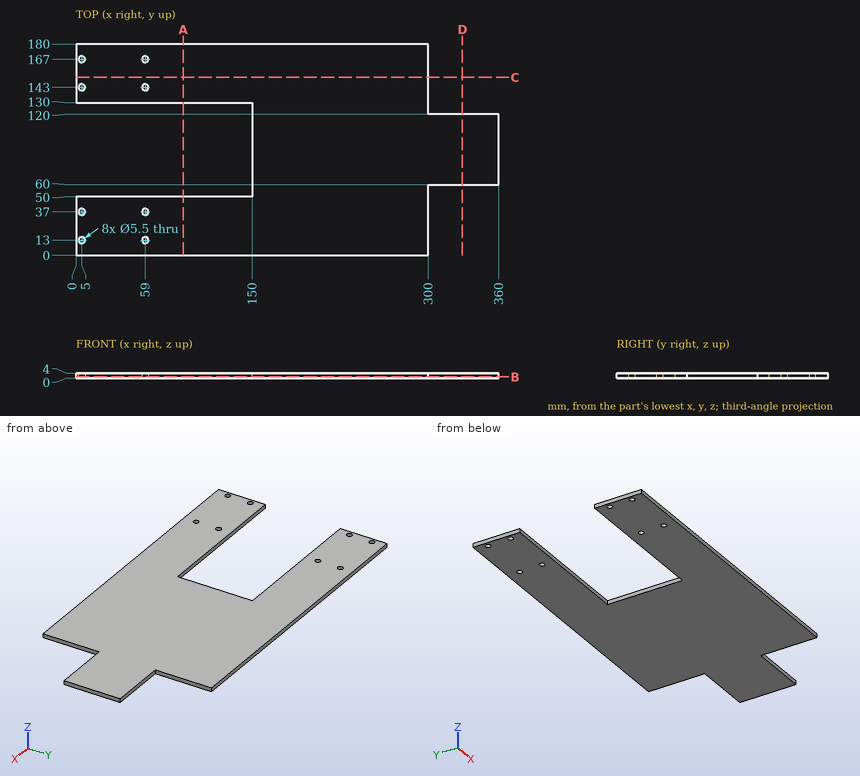
The figure shows three views and two pictorial views of one solid part (mm, origin at its lowest corner). Answer the questions. Give positions to 0.01 mm unless a question says otherwise; leave off trailing zeros. Write each loop counter-clockwise with the first axis right and the second up, starting at its lowest first coordinate (ties: lowest second). Pieces come first, ordered by that corner, then holes. Notation, with made-up numbers: (44.25, 70) - (96.25, 70) arc R6 cw to (96.25, 77) - close; hole circle Ø11 at (29.5, 47.25). An arc over 180 degrees is marked (long way). Use one line per item in the form item = value. Start each with the question number.
1) Consider line 1 along Y through (x, z) = (59, 0.85); line 2 along X through (y, z) = (143, 1.8); line 3 along Y through (x, z) = (18, 1). Determine where each line is inside the solid, lowest interval first. Write a range as from..to.
2) Find section C-C on y = 151.5. Determine the outline of the cut face in (x, z).
3) Find section D-D on x = 329. Determine the outline of the cut face in (y, z), plus the area to 3 significant figures.
4) Find section A-A on x = 91.5. Determine the outline of the cut face in (y, z), plus the area to 3 significant figures.
5) Find section B-B on z = 1. Count the separate pieces of the cut face and the enclosed holes in it, plus the area to 3 significant figures.
6) Flat-ended cylindrical pins translate along their axes: pin 1 Ø4.5 at (x, y) = (5, 143) entering from -Z; pin 2 Ø2 at (y, z) = (163.5, 1.5) entering from +X; pin 3 Ø1.2 at (x, z) = (338, 2) entering from -Y. Find the tip coordinate at first contact, or state that the pin passes through.
Geometry results:
q1.line_1 = 0..10.25, 15.75..34.25, 39.75..50, 130..140.25, 145.75..164.25, 169.75..180
q1.line_2 = 0..2.25, 7.75..56.25, 61.75..300
q1.line_3 = 0..50, 130..180
q2.outline = (0, 0) - (300, 0) - (300, 4) - (0, 4) - close
q3.outline = (60, 0) - (120, 0) - (120, 4) - (60, 4) - close
q3.area = 240 mm2
q4.outline = (0, 0) - (50, 0) - (50, 4) - (0, 4) - close; (130, 0) - (180, 0) - (180, 4) - (130, 4) - close
q4.area = 400 mm2
q5.separate_pieces = 1
q5.enclosed_holes = 8
q5.area = 45,400 mm2
q6.pin_1 = through
q6.pin_2 = 300
q6.pin_3 = 60
